```python
from build123d import *

# Parameters (mm, degrees)
SKETCH1_R                      = 29.75
BOSS_EXTRUDE1_DEPTH            = 23.2
SKETCH2_R                      = 6.3
CUT_EXTRUDE1_DEPTH             = 20.5
SKETCH3_R                      = 4.75
CUT_EXTRUDE2_DEPTH             = 2.7
CHAMFER1_SIZE                  = 0.5
CIRPATTERN1_COUNT              = 7
CIRPATTERN1_ANGLE              = 270
CIRPATTERN2_COUNT              = 4
CIRPATTERN3_COUNT              = 4
CUT_EXTRUDE3_DEPTH             = 5
FILLET1_R                      = 0.5
M3X0_5_TAPPED_HOLE4_D          = 2.5
M3X0_5_TAPPED_HOLE4_DEPTH      = 5
M3X0_5_TAPPED_HOLE4_TIP        = 0.751075774
M3X0_5_TAPPED_HOLE5_AT_2_COUNT = 2
M3X0_5_TAPPED_HOLE5_AT_2_PITCH = 10.774272925
CIRPATTERN4_COUNT              = 4


with BuildPart() as part:
    # Sketch1 → Boss-Extrude1 (new body)
    with BuildSketch(Plane(origin=(0, 0, 0), x_dir=(1, 0, 0), z_dir=(0, 1, 0))):
        Circle(SKETCH1_R)
    extrude(amount=BOSS_EXTRUDE1_DEPTH)

    # Sketch2 → Cut-Extrude1 (cut)
    with BuildSketch(Plane(origin=(0, 23.2, 0), x_dir=(1, 0, 0), z_dir=(0, 1, 0))):
        Circle(SKETCH2_R)
    extrude(amount=-CUT_EXTRUDE1_DEPTH, mode=Mode.SUBTRACT)

    # Sketch3 → Cut-Extrude2 (cut)
    with BuildSketch(Plane.XZ):
        Circle(SKETCH3_R)
    extrude(amount=-CUT_EXTRUDE2_DEPTH, mode=Mode.SUBTRACT)

    # Chamfer1
    chamfer1_edges = [part.edges().sort_by_distance(p)[0] for p in [
        (-29.75, 0, 0),
        (-29.75, 23.2, 0),
    ]]
    chamfer(chamfer1_edges, length=CHAMFER1_SIZE)

    # Sketch5 → M3x0.5 Tapped Hole1 (revolve, cut)
    with BuildSketch(Plane(origin=(0, 0, -22), x_dir=(0, 0, -1), z_dir=(1, 0, 0))):
        Polygon((0, 0), (0, 5.751075774), (1.25, 5), (1.25, 0), align=None)
    m3x0_5_tapped_hole1 = revolve(axis=Axis((0, -6.35, -22), (0, 1, 0)), mode=Mode.SUBTRACT)

    # CirPattern1: M3x0.5 Tapped Hole1 ×7 about axis
    cirpattern1_axis = Axis((0, 0, 0), (0, -1, 0))
    for i in range(1, CIRPATTERN1_COUNT):
        add(m3x0_5_tapped_hole1.rotate(cirpattern1_axis, i * CIRPATTERN1_ANGLE / (CIRPATTERN1_COUNT - 1)), mode=Mode.SUBTRACT)

    # Sketch7 → M3x0.5 Tapped Hole2 (revolve, cut)
    with BuildSketch(Plane(origin=(-8.838834765, 0, -8.838834765), x_dir=(0, 0, -1), z_dir=(1, 0, 0))):
        Polygon((0, 0), (0, 5.751075774), (1.25, 5), (1.25, 0), align=None)
    m3x0_5_tapped_hole2 = revolve(axis=Axis((-8.838834765, -6.35, -8.838834765), (0, 1, 0)), mode=Mode.SUBTRACT)

    # CirPattern2: M3x0.5 Tapped Hole2 ×4 about axis
    cirpattern2_axis = Axis((0, 0, 0), (0, 1, 0))
    for i in range(1, CIRPATTERN2_COUNT):
        add(m3x0_5_tapped_hole2.rotate(cirpattern2_axis, i * 360 / CIRPATTERN2_COUNT), mode=Mode.SUBTRACT)

    # Sketch9 → M3x0.5 Tapped Hole3 (revolve, cut)
    with BuildSketch(Plane(origin=(-15, 0, 0), x_dir=(0, 0, -1), z_dir=(1, 0, 0))):
        Polygon((0, 0), (0, 5.751075774), (1.25, 5), (1.25, 0), align=None)
    m3x0_5_tapped_hole3 = revolve(axis=Axis((-15, -6.35, 0), (0, 1, 0)), mode=Mode.SUBTRACT)

    # CirPattern3: M3x0.5 Tapped Hole3 ×4 about axis
    cirpattern3_axis = Axis((0, 0, 0), (0, 1, 0))
    for i in range(1, CIRPATTERN3_COUNT):
        add(m3x0_5_tapped_hole3.rotate(cirpattern3_axis, i * 360 / CIRPATTERN3_COUNT), mode=Mode.SUBTRACT)

    # Sketch10 → Cut-Extrude3 (cut)
    with BuildSketch(Plane.XZ):
        Polygon((-20.11656159, -13.815821112), (-13.045493778, -20.886888923), (-15.873920903, -23.715316048), (-22.944988715, -16.644248236), align=None)
    extrude(amount=-CUT_EXTRUDE3_DEPTH, mode=Mode.SUBTRACT)

    # Fillet1
    fillet1_edges = [part.edges().sort_by_distance(p)[0] for p in [
        (-22.944988715, 2.5, -16.644248236),
        (-20.11656159, 2.5, -13.815821112),
        (-13.045493778, 2.5, -20.886888923),
        (-15.873920903, 2.5, -23.715316048),
    ]]
    fillet(fillet1_edges, radius=FILLET1_R)

    # M3x0.5 Tapped Hole4
    with Locations(Plane(origin=(0, 23.2, 0), x_dir=(1, 0, 0), z_dir=(0, 1, 0))):
        with Locations((-17, 17), (-17, -17), (17, -17), (17, 17)):
            Hole(M3X0_5_TAPPED_HOLE4_D / 2, depth=M3X0_5_TAPPED_HOLE4_DEPTH)
            with Locations((0, 0, -(M3X0_5_TAPPED_HOLE4_DEPTH + M3X0_5_TAPPED_HOLE4_TIP / 2))):  # 118° drill point
                Cone(0, M3X0_5_TAPPED_HOLE4_D / 2, M3X0_5_TAPPED_HOLE4_TIP, mode=Mode.SUBTRACT)

    # Sketch14 → M3x0.5 Tapped Hole5 (revolve, cut)
    with BuildSketch(Plane(origin=(12.5, 23.2, 0), x_dir=(0, 0, 1), z_dir=(1, 0, 0))):
        Polygon((0, 0), (0, 5.751075774), (1.25, 5), (1.25, 0), align=None)
    m3x0_5_tapped_hole5 = revolve(axis=Axis((12.5, 29.55, 0), (0, -1, 0)), mode=Mode.SUBTRACT)

    # M3x0.5 Tapped Hole5 at 2: M3x0.5 Tapped Hole5 ×2
    with Locations(*[Vector(-0.175733276, 0, -0.984437817) * (i * M3X0_5_TAPPED_HOLE5_AT_2_PITCH) for i in range(1, M3X0_5_TAPPED_HOLE5_AT_2_COUNT)]):
        add(m3x0_5_tapped_hole5, mode=Mode.SUBTRACT)

    # CirPattern4: M3x0.5 Tapped Hole5 ×4 about axis
    cirpattern4_axis = Axis((0, 0, 0), (0, 1, 0))
    for i in range(1, CIRPATTERN4_COUNT):
        add(m3x0_5_tapped_hole5.rotate(cirpattern4_axis, i * 360 / CIRPATTERN4_COUNT), mode=Mode.SUBTRACT)

    # CirPattern4 copy 1 sketch → CirPattern4 copy 1 (revolve, cut)
    with BuildSketch(Plane(origin=(-10.606601718, 23.2, -10.606601718), x_dir=(1, 0, 0), z_dir=(0, 0, -1))):
        Polygon((0, 0), (0, 5.751075774), (1.25, 5), (1.25, 0), align=None)
    revolve(axis=Axis((-10.606601718, 29.55, -10.606601718), (0, -1, 0)), mode=Mode.SUBTRACT)

    # CirPattern4 copy 2 sketch → CirPattern4 copy 2 (revolve, cut)
    with BuildSketch(Plane(origin=(-10.606601718, 23.2, 10.606601718), x_dir=(0, 0, -1), z_dir=(-1, 0, 0))):
        Polygon((0, 0), (0, 5.751075774), (1.25, 5), (1.25, 0), align=None)
    revolve(axis=Axis((-10.606601718, 29.55, 10.606601718), (0, -1, 0)), mode=Mode.SUBTRACT)

    # CirPattern4 copy 3 sketch → CirPattern4 copy 3 (revolve, cut)
    with BuildSketch(Plane(origin=(10.606601718, 23.2, 10.606601718), x_dir=(-1, 0, 0), z_dir=(0, 0, 1))):
        Polygon((0, 0), (0, 5.751075774), (1.25, 5), (1.25, 0), align=None)
    revolve(axis=Axis((10.606601718, 29.55, 10.606601718), (0, -1, 0)), mode=Mode.SUBTRACT)


solid = part.part
```
Verification items for the finished model (mm, model axes). A direction names the side the tool comes from. Coordinates: 2 decimals unless noted, no trailing zeros. Put each result on its own line as item: value.
1. Thickness scan on line 1 (Z direction, x = 0, y = 19.35); line 2 (Z direction, x = -16.5, y = 2.75); line 3 (X direction, y = 4.5, z = 9). Record the ranges inside material, lowest first.
Result set:
line 1: z = -29.75 to -13.75, -11.25 to -6.3, 6.3 to 11.25, 13.75 to 29.75
line 2: z = -24.76 to -23.09, -17.43 to 14.74, 16.38 to 24.76
line 3: x = -28.36 to -10.08, -7.6 to 7.6, 10.08 to 28.36
2. Gauge pin test, flat ends, axial feed: P1, Ø3, axis at x = 12.5, z = 0, coming from the +Y side; P2, Ø3, axis at x = -20.5, y = 14, coming from the +Z side; P3, Ø4, axis at x = -3, z = 1.5, coming from the +Y side; P4, Ø12, axis at x = 3.5, y = 7, coming from the +Z side. Record the tip position at first contact, or that the pin passes through.
Result set:
P1: stops at y = 23.2
P2: stops at z = 22.89
P3: stops at y = 2.7
P4: stops at z = 29.75
3. Tool access check on faces 3 (the face through (0.16, 20.74, 11.26)), 4 (the face through (0.672, 2.465, -16.054)). Record the directions out of +Z, -Z, +X, -X, +Y, -Y that give a thin tool (end or side, any length) a straight path to the whole face; none if there is none.
Result set:
face 3: +Y
face 4: -Y
4. Mould release check, pull along X, two halves, no side actions. Record for faces 1 (the face through (15.993, 11.445, -25.085)), 2 (the face through (0.08, 5.62, -22.2)): pulls with the +X half, pulls with the -X half, needs draft (parallel to the pull), parting line crosses it, or undercut.
Result set:
face 1: parting line crosses it
face 2: undercut
5. Section check A-A, the plane y = 3.75. Give the number of separate pieces and of enclosed holes in the cut face, then the cut area to 3 significant figures.
Result set:
separate pieces: 1
enclosed holes: 17
area: 2,540 mm^2
